Read the model definition and answer for the solid it produces. Units are mm, in the model's axes. Coordinates: 2 decimals unless noted, no trailing zeros. Write each loop counter-clockwise with the first axis right and the second up, starting at its lowest first coordinate (ties: lowest second). Pieces come first, ordered by that corner, then holes. Notation, with made-up numbers: M -15.5,67.5 L 40.5,67.5 A14 cw 40.5,76.5 Z; hole C 2,8 d7. An arc over 180 degrees is marked long. Write item = value, one per line.
Autodesk Inventor part; units mm, degrees
ref_plane "YZ Plane" through (0, 0, 0) normal (1, 0, 0) x (0, 1, 0)
ref_plane "XZ Plane" through (0, 0, 0) normal (0, 1, 0) x (-1, 0, 0)
ref_plane "XY Plane" through (0, 0, 0) normal (0, 0, 1) x (1, 0, 0)
sketch "Boceto1" plane through (0, 0, 0) normal (0, 1, 0) x (-1, 0, 0)
  line L0 (27, 411.5) -> (0, 411.5)
  line L1 (0, 411.5) -> (0, -411.5)
  line L2 (0, -411.5) -> (27, -411.5)
  line L3 (27, -411.5) -> (27, 411.5)
  line L4 (0, 0) -> (280.3389, 0)
  dimension "d0" = 823
  dimension "d1" = 27
extrude "Extrusión1" add sketch "Boceto1" along normal blind 3
sketch "Boceto2" plane through (0, 3, 0) normal (0, 1, 0) x (1, 0, 0)
  line L0 (0, -441.5) -> (3, -441.5)
  line L1 (3, -441.5) -> (3, 441.5)
  line L2 (3, 441.5) -> (0, 441.5)
  line L3 (0, 441.5) -> (0, -441.5)
  line L4 (0, 0) -> (-318.7817, 0)
  point P0 (0, -411.5)
  dimension "d4" = 883
  dimension "d5" = 3
extrude "Extrusión2" add sketch "Boceto2" against normal blind 30
sketch "Boceto3" plane through (3, 3, 441.5) normal (1, 0, 0) x (0, 0, -1)
  line L0 (883, -30) -> (0, -30)
  line L1 (441.5, -30) -> (441.5, 0)
  line L2 (853, 0) -> (30, 0)
  line L3 (456.5, -30) -> (426.5, -30)
  line L4 (426.5, -30) -> (426.5, 0)
  line L5 (426.5, 0) -> (456.5, 0)
  line L6 (456.5, 0) -> (456.5, -30)
  line L7 (0, 0) -> (883, 0)
  line L8 (30, -3) -> (853, -3)
  point P0 (441.5, -3)
  point P1 (456.5, -3)
  point P2 (426.5, -3)
  dimension "d8" = 30
extrude "Extrusión3" cut sketch "Boceto3" against normal blind 10 contours L0 L1 L8 L6 | L0 L4 L8 L1
fillet "Empalme1" radius 2 2 edges at (1.5, -27, 15) (1.5, -27, -15)
properties part number "A_3030_INT"
Item 1: Flat-ended cylindrical pins translate along their axes: pin 1 (5 mm diameter, centred on x = -16.5, z = -326.5, fed in from -Y); pin 2 (2.5 mm diameter, centred on x = -13, y = 1, fed in from -Z); pin 3 (2.5 mm diameter, centred on x = -9.5, y = 2, fed in from +Z). Find the tip coordinate at first contact, or state that the pin passes through.
Worked answers:
pin_1 = 0
pin_2 = -411.5
pin_3 = 411.5
Item 2: Find section C-C (x = -13.25). Determine the outline of the cut face in (y, z), and give its area (3 significant figures).
Worked answers:
outline = M 0,-411.5 L 3,-411.5 L 3,411.5 L 0,411.5 Z
area = 2,470 mm²
Item 3: Find section B-B (z = 259.5). Determine the outline of the cut face in (x, y), and give its area (3 significant figures).
Worked answers:
outline = M -27,0 L 0,0 L 0,-27 L 3,-27 L 3,3 L -27,3 Z
area = 171 mm²
Item 4: Find section A-A (y = -5). Determine the outline of the cut face in (x, z).
Worked answers:
outline = M 0,-441.5 L 3,-441.5 L 3,-15 L 0,-15 Z; M 0,15 L 3,15 L 3,441.5 L 0,441.5 Z
Item 5: Consider line 1 along X through (y, z) = (-25.5, 54); line 2 along Z through (x, y) = (-6.75, 0.5). Determine where each line is inside the solid, lowest interval first. Write a range as from..to.
Worked answers:
line_1 = 0..3
line_2 = -411.5..411.5
